For this review, use the dimensioned drawing (mm, ordinates from the lowest corner) and the shaded views. A direction names the side the tool comes from. Coordinates: 2 decimals unless noted, no trailing zeros. Order: outer loops, then holes, each group sorted by start corner. A loop starts at its lowest first (then second) coordinate and runs counter-clockwise, first axis right, second up. Notation, with made-up numbers: (-9, 14) -> (20, 14) arc R26 ccw to (20, 52) -> close; hole circle Ø7 at (-37.75, 5.25). An arc over 180 degrees is marked (long way). Return JSON: item names as keys, results as strings. Group by question number.
Item 1: Take a section at D-D (z = 42). Write out the cut boundary in (x, y).
Item 2: Take a section at C-C (x = 103). Write out the cut boundary in (y, z).
Item 3: Insertion check: pin 1 (1 mm diameter, centred on x = 107.5, z = 15.5, fed in from +Y); pin 2 (5 mm diameter, centred on x = 110, z = 38, fed in from +Y); pin 3 (3.5 mm diameter, centred on y = 9, z = 31, fed in from +X). Each pin has a flat end and moves straight along its axis. Give the tip position at first contact, or say it passes through.
Item 4: Take a section at B-B (y = 9.5). Write out the cut boundary in (x, z).
Item 5: For line 1 along X through (y, z) = (5.25, 62); line 2 along X through (y, z) = (12.75, 37.5) (1 decimal); line 3 along Z through (x, y) = (98.5, 8.5) (1 decimal), list the stretches that pass through material, from the lowest coordinate up.
Item 6: Machinability: for the marked faces 4, 5 and 6, which of the approach directions +Z, -Z, +X, -X, +Y, -Y give a long, thin tool a straight path to every point of the face, cutting with its end or side? Answer none if there is none.
Item 7: Draft analysis for pull direction Z (two halves, no side actions). For the marked faces 1, 2 and 3, state which applies: +Z half, -Z half, draft (parallel to the pull), parting line (faces both ways), or undercut.
Item 8: Take a section at A-A (z = 55.5). Write out the cut boundary in (x, y), then the cut area to 3 significant figures.
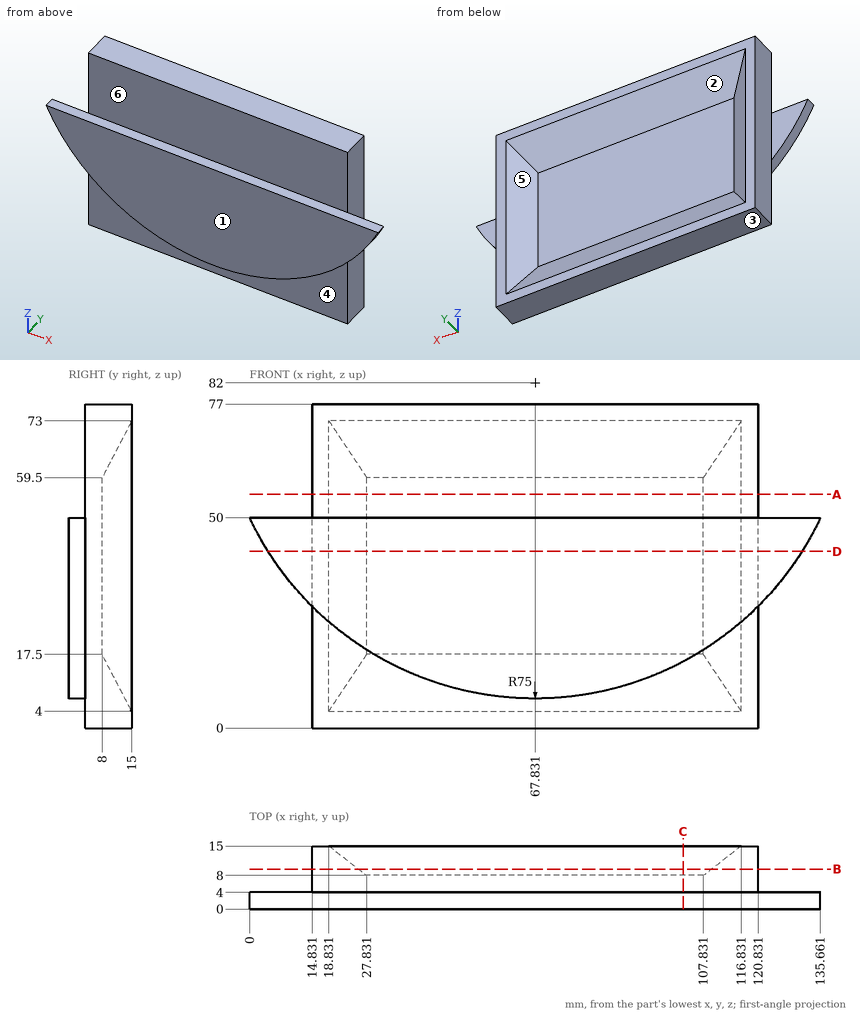
Findings below:
{
 "1": {"outline": "(4.39, 0) -> (131.27, 0) -> (131.27, 4) -> (120.83, 4) -> (120.83, 15) -> (116.83, 15) -> (107.83, 8) -> (27.83, 8) -> (18.83, 15) -> (14.83, 15) -> (14.83, 4) -> (4.39, 4) -> close"},
 "2": {"outline": "(0, 15.76) -> (4, 15.76) -> (4, 0) -> (15, 0) -> (15, 4) -> (8, 17.5) -> (8, 59.5) -> (15, 73) -> (15, 77) -> (4, 77) -> (4, 50) -> (0, 50) -> close"},
 "3": {"pin 1": "stops at y = 9.3", "pin 2": "stops at y = 11.63", "pin 3": "stops at x = 120.83"},
 "4": {"outline": "(14.83, 0) -> (120.83, 0) -> (120.83, 77) -> (14.83, 77) -> close; hole (25.9, 14.61) -> (109.76, 14.61) -> (109.76, 62.39) -> (25.9, 62.39) -> close"},
 "5": {"line 1": "x = 14.83 to 120.83", "line 2": "x = 14.8 to 21.7, 113.9 to 120.8", "line 3": "z = 0 to 16.5, 60.5 to 77"},
 "6": {"face 4": "-Z, -Y", "face 5": "+Y", "face 6": "+Z, +X, -X, -Y"},
 "7": {"face 1": "draft", "face 2": "undercut", "face 3": "-Z half"},
 "8": {"outline": "(14.83, 4) -> (120.83, 4) -> (120.83, 15) -> (116.83, 15) -> (107.83, 8) -> (27.83, 8) -> (18.83, 15) -> (14.83, 15) -> close", "area": "543 mm2"}
}
